Here's how the part is built. I have some questions about the finished solid (model axes, mm). Face numbers are marked on the shaded views. Round coordinates to 2 decimals unless told otherwise and drop trailing zeros. Write each loop counter-clockwise with the first axis right and the second up, starting at its lowest first coordinate (ties: lowest second). Pieces come first, ordered by that corner, then holes. Notation, with made-up numbers: (48.5, 14.5) -> (70.5, 14.5) arc R28 ccw to (70.5, 40.5) -> close; hole circle Ø5 at (-10.5, 48). An arc over 180 degrees is marked (long way). Answer in a Markdown table with one row per item.
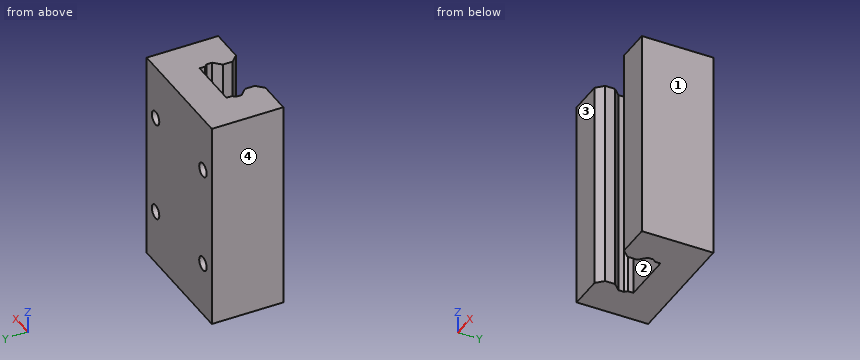
from build123d import *

# Parameters (mm, degrees)
BOSS_EXTRUDE1_DEPTH = 75
SKETCH2_R           = 2.5
CUT_EXTRUDE1_DEPTH  = 6


with BuildPart() as part:
    # Sketch1 → Boss-Extrude1 (new body)
    with BuildSketch(Plane.XY):
        Polygon((-22, 0), (22, 0), (22, -25.4), (10, -25.4), (7.5, -22.9), (7.5, -19.4), (10, -16.9), (10, -14.9), (9.1, -14), (9.1, -12), (-9.1, -12), (-9.1, -14), (-10, -14.9), (-10, -16.9), (-7.5, -19.4), (-7.5, -22.9), (-10, -25.4), (-22, -25.4), align=None)
    extrude(amount=-BOSS_EXTRUDE1_DEPTH)

    # Sketch2 → Cut-Extrude1 (cut)
    with BuildSketch(Plane(origin=(0, 0, 0), x_dir=(1, 0, 0), z_dir=(0, 1, 0))):
        with Locations(Location((-16, 55.5, 0), (0, 0, 270))):
            Circle(SKETCH2_R)
        with Locations(Location((-16, 19.5, 0), (0, 0, 270))):
            Circle(SKETCH2_R)
        with Locations(Location((16, 55.5, 0), (0, 0, 270))):
            Circle(SKETCH2_R)
        with Locations(Location((16, 19.5, 0), (0, 0, 270))):
            Circle(SKETCH2_R)
    extrude(amount=-CUT_EXTRUDE1_DEPTH, mode=Mode.SUBTRACT)


solid = part.part
1) I want a section at D-D, the plane z = -19.5. List the corners of the cut face in (x, y) for me, and give its area (3 significant figures).
Response:
| item | result |
|---|---|
| outline | (-22, -25.4) -> (-10, -25.4) -> (-7.5, -22.9) -> (-7.5, -19.4) -> (-10, -16.9) -> (-10, -14.9) -> (-9.1, -14) -> (-9.1, -12) -> (9.1, -12) -> (9.1, -14) -> (10, -14.9) -> (10, -16.9) -> (7.5, -19.4) -> (7.5, -22.9) -> (10, -25.4) -> (22, -25.4) -> (22, 0) -> (18.5, 0) -> (18.5, -6) -> (13.5, -6) -> (13.5, 0) -> (-13.5, 0) -> (-13.5, -6) -> (-18.5, -6) -> (-18.5, 0) -> (-22, 0) -> close |
| area | 824 mm^2 |
2) I want a section at B-B, the plane z = -7.5. List the corners of the cut face in (x, y) for me.
Response:
| item | result |
|---|---|
| outline | (-22, -25.4) -> (-10, -25.4) -> (-7.5, -22.9) -> (-7.5, -19.4) -> (-10, -16.9) -> (-10, -14.9) -> (-9.1, -14) -> (-9.1, -12) -> (9.1, -12) -> (9.1, -14) -> (10, -14.9) -> (10, -16.9) -> (7.5, -19.4) -> (7.5, -22.9) -> (10, -25.4) -> (22, -25.4) -> (22, 0) -> (-22, 0) -> close |
3) I want a section at A-A, the plane x = 16. List the corners of the cut face in (y, z) for me, and give its area (4 significant figures).
Response:
| item | result |
|---|---|
| outline | (-25.4, -75) -> (0, -75) -> (0, -58) -> (-6, -58) -> (-6, -53) -> (0, -53) -> (0, -22) -> (-6, -22) -> (-6, -17) -> (0, -17) -> (0, 0) -> (-25.4, 0) -> close |
| area | 1,845 mm^2 |
4) I want a section at C-C, the plane y = -1.25. List the corners of the cut face in (x, z) for me.
Response:
| item | result |
|---|---|
| outline | (-22, -75) -> (22, -75) -> (22, 0) -> (-22, 0) -> close; hole circle Ø5 at (-16, -55.5); hole circle Ø5 at (-16, -19.5); hole circle Ø5 at (16, -55.5); hole circle Ø5 at (16, -19.5) |
5) For pin 1 (4 mm diameter, centred on x = -16, z = -55.5, fed in from +Y); pin 2 (5.5 mm diameter, centred on x = 0, z = -46, fed in from -Y), each with a flat end and sliding along its axis, tell me the tip position at first contact or that it passes through.
Response:
| item | result |
|---|---|
| pin 1 | stops at y = -6 |
| pin 2 | stops at y = -12 |
6) We'd pull the mould along X, two halves only. Please class the marked faces 1, 2, 3 and 4: +X half, -X half, draft (parallel to the pull), parting line (faces both ways), or undercut.
Response:
| item | result |
|---|---|
| face 1 | +X half |
| face 2 | undercut |
| face 3 | draft |
| face 4 | -X half |
7) I need wall thicknesses on line 1 (X direction, y = -4.55, z = -55.5); line 2 (X direction, y = -19.75, z = -57.5); line 3 (Y direction, x = -9.5, z = -45). Which ranges of each line are inside material? Lowest first, please. Write a range as [from, to].
Response:
| item | result |
|---|---|
| line 1 | x = [-22, -18.5], [-13.5, 13.5], [18.5, 22] |
| line 2 | x = [-22, -7.5], [7.5, 22] |
| line 3 | y = [-24.9, -17.4], [-14.4, 0] |
